CAD build for the part. Positions are in the model's coordinates, mm. A direction names the side the tool comes from. Coordinates: 2 decimals unless noted, no trailing zeros. Loops run counter-clockwise (first coordinate to the right, second up) from the corner with the lowest first, then second, coordinate; pieces in that order, holes last. Notation, with made-up numbers: (-19, 78) -> (12, 78) arc R23 cw to (12, 95) -> close; hole circle Ø11 at (17, 46.25). An arc over 180 degrees is marked (long way). Return JSON: item names as keys, results as strings. Group by question number.
(1) Saw through at B-B on x = 0. Write the cut outline in (y, z).
(2) Mould opens along X. For faces 1 (the face through (0, 0, 21)), 2 (the face through (-10, -39, 4)), 3 (the face through (-5.46, -35.17, 6.04)) say: pulls with the +X half, pulls with the -X half, needs draft (parallel to the pull), parting line crosses it, or undercut.
(3) Tool access for faces 4 (the face through (-0.534, 4.065, 3.451)), 5 (the face through (0, 0, 0)), 6 (the face through (24.994, -0.53, 16.493)), 7 (the face through (18, -21, 14)): list every direction of +Z, -Z, +X, -X, +Y, -Y with a clear straight run to the whole face (end or side of a thin tool).
(4) Saw through at A-A on z = 8. Write the cut outline in (x, y), then the cut area to 3 significant figures.
(5) Saw through at C-C on z = 1. Write the cut outline in (x, y), then the cut area to 3 significant figures.
(6) Flat gauge pins, fed straight in: pin 1 Ø10 at (y, z) = (14.5, 12.5) entering from +X; pin 2 Ø1 at (x, y) = (-25.5, 10.5) entering from -Z; pin 3 Ø5 at (y, z) = (-28, 15) entering from -X. Where does each tip first touch, or does it go through?
(7) Probe L1, parallel to Z at x = 29, y = -1; L2, parallel to Z at x = 6, y = 14.5; L3, parallel to Z at x = -9, y = -31.5. List the from-to ranges inside material, lowest first.
```python
from build123d import *

# Parameters (mm, degrees)
SKETCH1_R               = 4.1
BOSS_EXTRUDE1_DEPTH     = 7
SKETCH2_R               = 6.25
BOSS_EXTRUDE2_DEPTH     = 2
SKETCH3_R               = 35
BOSS_EXTRUDE3_DEPTH     = 5
SKETCH4_R               = 25
BOSS_EXTRUDE4_DEPTH     = 5
SKETCH5_R               = 30
BOSS_EXTRUDE5_DEPTH     = 2
FILLET1_R               = 2
FILLET2_R               = 2
SKETCH6_R               = 1.5
CUT_EXTRUDE1_DEPTH      = 36
CUT_EXTRUDE1_DEPTH_BACK = 36
BOSS_EXTRUDE6_DEPTH     = 10
SKETCH9_R               = 1.75
CUT_EXTRUDE2_DEPTH      = 1
CUT_EXTRUDE2_DEPTH_BACK = 23
SKETCH10_R              = 3.5
CUT_EXTRUDE3_DEPTH      = 6


with BuildPart() as part:
    # Sketch1 → Boss-Extrude1 (new body)
    with BuildSketch(Plane.XY):
        Circle(SKETCH1_R)
    extrude(amount=BOSS_EXTRUDE1_DEPTH)

    # Sketch2 → Boss-Extrude2 (add)
    with BuildSketch(Plane.XY.offset(7)):
        Circle(SKETCH2_R)
    extrude(amount=BOSS_EXTRUDE2_DEPTH)

    # Sketch3 → Boss-Extrude3 (add)
    with BuildSketch(Plane.XY.offset(9)):
        Circle(SKETCH3_R)
    extrude(amount=BOSS_EXTRUDE3_DEPTH)

    # Sketch4 → Boss-Extrude4 (add)
    with BuildSketch(Plane.XY.offset(14)):
        Circle(SKETCH4_R)
    extrude(amount=BOSS_EXTRUDE4_DEPTH)

    # Sketch5 → Boss-Extrude5 (add)
    with BuildSketch(Plane.XY.offset(19)):
        Circle(SKETCH5_R)
    extrude(amount=BOSS_EXTRUDE5_DEPTH)

    # Fillet1
    fillet1_edges = [part.edges().sort_by_distance(p)[0] for p in [
        (-25, 0, 19),
    ]]
    fillet(fillet1_edges, radius=FILLET1_R)

    # Fillet2
    fillet2_edges = [part.edges().sort_by_distance(p)[0] for p in [
        (-25, 0, 14),
    ]]
    fillet(fillet2_edges, radius=FILLET2_R)

    # Sketch6 → Cut-Extrude1 (cut, two sides)
    with BuildSketch(Plane(origin=(0, 0, 0), x_dir=(1, 0, 0), z_dir=(0, 1, 0))) as cut_extrude1_sk:
        with Locations((0.008646323, -16.5)):
            Circle(SKETCH6_R)
    extrude(amount=CUT_EXTRUDE1_DEPTH, mode=Mode.SUBTRACT)
    extrude(cut_extrude1_sk.sketch, amount=-CUT_EXTRUDE1_DEPTH_BACK, mode=Mode.SUBTRACT)

    # Sketch7 → Boss-Extrude6 (add)
    with BuildSketch(Plane(origin=(0, 0, 9), x_dir=(-1, 0, 0), z_dir=(0, 0, -1))):
        with BuildLine():
            Line((35, 0), (27, 0))
            ThreePointArc((27, 0), (15.149257408, -22.349496639), (-10, -25.079872408))
            Line((-10, -25.079872408), (-10, -43.735334875))
            Line((-10, -43.735334875), (10, -43.735334875))
            Line((10, -43.735334875), (10, -33.735334875))
            Line((10, -33.735334875), (10, -33.541019662))
            ThreePointArc((10, -33.541019662), (28.062430401, -20.916500663), (35, 0))
        make_face()
    extrude(amount=BOSS_EXTRUDE6_DEPTH)

    # Sketch9 → Cut-Extrude2 (cut, two sides)
    with BuildSketch(Plane(origin=(0, 0, -1), x_dir=(-1, 0, 0), z_dir=(0, 0, -1))) as cut_extrude2_sk:
        with Locations((5, -38.638177269)):
            Circle(SKETCH9_R)
        with Locations((-5, -38.638177269)):
            Circle(SKETCH9_R)
    extrude(amount=CUT_EXTRUDE2_DEPTH, mode=Mode.SUBTRACT)
    extrude(cut_extrude2_sk.sketch, amount=-CUT_EXTRUDE2_DEPTH_BACK, mode=Mode.SUBTRACT)

    # Sketch10 → Cut-Extrude3 (cut)
    with BuildSketch(Plane.XY.offset(9)):
        with Locations((-5, -38.638177269)):
            Circle(SKETCH10_R)
        with Locations((5, -38.638177269)):
            Circle(SKETCH10_R)
    extrude(amount=-CUT_EXTRUDE3_DEPTH, mode=Mode.SUBTRACT)


solid = part.part
```
Geometry results:
{
 "1": {"outline": "(-43.74, -1) -> (-27, -1) -> (-27, 9) -> (-6.25, 9) -> (-6.25, 7) -> (-4.1, 7) -> (-4.1, 0) -> (4.1, 0) -> (4.1, 7) -> (6.25, 7) -> (6.25, 9) -> (35, 9) -> (35, 14) -> (27, 14) arc R2 cw to (25.27, 15) -> (-25.27, 15) arc R2 cw to (-27, 14) -> (-35, 14) -> (-35, 9) -> (-43.74, 9) -> close; (-30, 19) -> (-27, 19) arc R2 cw to (-25.27, 18) -> (25.27, 18) arc R2 cw to (27, 19) -> (30, 19) -> (30, 21) -> (-30, 21) -> close"},
 "2": {"face 1": "needs draft", "face 2": "pulls with the -X half", "face 3": "undercut"},
 "3": {"face 4": "-Z", "face 5": "-Z, +X, +Y", "face 6": "+X", "face 7": "none"},
 "4": {"outline": "(-35, 0) arc R35 ccw to (-10, -33.54) -> (-10, -43.74) -> (10, -43.74) -> (10, -25.08) arc R27 cw to (-27, 0) -> close; circle Ø12.5 at (0, 0); hole circle Ø7 at (-5, -38.64); hole circle Ø7 at (5, -38.64)", "area": "701 mm²"},
 "5": {"outline": "(-35, 0) arc R35 ccw to (-10, -33.54) -> (-10, -43.74) -> (10, -43.74) -> (10, -25.08) arc R27 cw to (-27, 0) -> close; circle Ø8.2 at (0, 0); hole circle Ø3.5 at (-5, -38.64); hole circle Ø3.5 at (5, -38.64)", "area": "689 mm²"},
 "6": {"pin 1": "x = 33.69", "pin 2": "z = 9", "pin 3": "x = -23.75"},
 "7": {"L1": "9 to 14, 19 to 21", "L2": "9 to 21", "L3": "-1 to 14"}
}
